Solid Edge part; units mm, degrees
sketch "Sketch1" plane through (0, 0, 0) normal (0, 0, 1) x (1, 0, 0)
  line L0 (-23.7579, 34.8421) -> (-23.7579, -27.1579)
  line L1 (-23.7579, -27.1579) -> (38.2421, -27.1579)
  line L2 (38.2421, -27.1579) -> (38.2421, 34.8421)
  line L3 (38.2421, 34.8421) -> (-23.7579, 34.8421)
  line L4 (-27.7579, 38.8421) -> (-27.7579, -31.1579)
  line L5 (-27.7579, -31.1579) -> (42.2421, -31.1579)
  line L6 (42.2421, -31.1579) -> (42.2421, 38.8421)
  line L7 (42.2421, 38.8421) -> (-27.7579, 38.8421)
  dimension "D1" = 42.2421
  dimension "D2" = 42.2421
  dimension "D3" = 38.2421
extrude "Protrusion1" add sketch "Sketch1" along normal blind 125
hole "Hole_1" at (-17.7579, 38.8421, 62.5) direction (0, -1, 0) diameter 7 end up to next
hole "Hole1" at (-17.7579, 38.8421, 25) direction (0, -1, 0) diameter 7 end up to next
hole "Hole2" at (-17.7579, 38.8421, 100) direction (0, -1, 0) diameter 7 end up to next
hole "Hole_4" at (-12.7579, -31.1579, 62.5) direction (0, 1, 0) diameter 7 end up to next
hole "Hole3" at (-12.7579, -31.1579, 100) direction (0, 1, 0) diameter 7 end up to next
hole "Hole4" at (27.2421, -31.1579, 100) direction (0, 1, 0) diameter 7 end up to next
hole "Hole5" at (27.2421, -31.1579, 62.5) direction (0, 1, 0) diameter 7 end up to next
hole "Hole6" at (27.2421, -31.1579, 25) direction (0, 1, 0) diameter 7 end up to next
hole "Hole7" at (-12.7579, -31.1579, 25) direction (0, 1, 0) diameter 7 end up to next
Geometry check sheet. Reference: the model listing, model coordinates, mm. A direction names the side the tool comes from. Coordinates: 2 decimals unless noted, no trailing zeros. Order: outer loops, then holes, each group sorted by start corner. A loop starts at its lowest first (then second) coordinate and runs counter-clockwise, first axis right, second up. Notation, with made-up numbers: M 74.25,28 L 109.25,28 A33 cw 109.25,63 Z; hole C 75,11 d5. An arc over 180 degrees is marked long. Answer as a JSON object with one key per item and string values.
Q1. Release check for a two-part mould opening along X. For faces 4 (the flat face through (-27.758, 4, 62)), 5 (the cylindrical face through (-11.71, -29.19, 96.66)), 6 (the flat face through (8, 38.842, 62)) record: released by +X, released by -X, zero draft, split by the parting line, or undercut.
Results are:
{"face 4": "released by -X", "face 5": "undercut", "face 6": "zero draft"}
Q2. Cross-section at A-A on z = 62.5. Record the cut outline in (x, y), and give its area (3 significant figures).
Results are:
{"outline": "M -27.76,-31.16 L -16.26,-31.16 L -16.26,-27.16 L -23.76,-27.16 L -23.76,34.84 L -21.26,34.84 L -21.26,38.84 L -27.76,38.84 Z; M -14.26,34.84 L 38.24,34.84 L 38.24,-27.16 L 30.74,-27.16 L 30.74,-31.16 L 42.24,-31.16 L 42.24,38.84 L -14.26,38.84 Z; M -9.26,-31.16 L 23.74,-31.16 L 23.74,-27.16 L -9.26,-27.16 Z", "area": "972 mm²"}
Q3. Cross-section at B-B on y = -11.5. Record the cut outline in (x, z), and give its area (4 significant figures).
Results are:
{"outline": "M -27.76,0 L -23.76,0 L -23.76,125 L -27.76,125 Z; M 38.24,0 L 42.24,0 L 42.24,125 L 38.24,125 Z", "area": "1,000 mm²"}
Q4. Cross-section at D-D on z = 75.5. Record the cut outline in (x, y), and give its area (3 significant figures).
Results are:
{"outline": "M -27.76,-31.16 L 42.24,-31.16 L 42.24,38.84 L -27.76,38.84 Z; hole M -23.76,-27.16 L 38.24,-27.16 L 38.24,34.84 L -23.76,34.84 Z", "area": "1,060 mm²"}
Q5. Depth check by flat-ended pin: pin 1 Ø6.5 at (x, z) = (27.24, 62.5) entering from -Y; pin 2 Ø4 at (x, z) = (-17.76, 25) entering from +Y. Enter the tip coordinate at first touch or a pass-through.
Results are:
{"pin 1": "stops at y = 34.84", "pin 2": "stops at y = -27.16"}
Q6. Tool access check on faces 1 (the flat face through (38.242, 3, 62)), 2 (the cylindrical face through (-17.604, 36.87, 59.003)), 3 (the cylindrical face through (-9.807, -29.186, 23.118)). Record the directions out of +Z, -Z, +X, -X, +Y, -Y that give a thin tool (end or side, any length) a straight path to the whole face; none if there is none.
Results are:
{"face 1": "+Z, -Z", "face 2": "+Y", "face 3": "-Y"}
Q7. Scan lines: line 1 (X direction, y = -29.6, z = 100); line 2 (X direction, y = -10.5, z = 63); line 3 (Y direction, x = -4.5, z = 18). Record each from-to range of solid material in increasing order.
Results are:
{"line 1": "x = -27.76 to -16.26, -9.26 to 23.74, 30.74 to 42.24", "line 2": "x = -27.76 to -23.76, 38.24 to 42.24", "line 3": "y = -31.16 to -27.16, 34.84 to 38.84"}
Q8. Cross-section at C-C on x = 7.5. Record the cut outline in (y, z), and give its area (3 significant figures).
Results are:
{"outline": "M -31.16,0 L -27.16,0 L -27.16,125 L -31.16,125 Z; M 34.84,0 L 38.84,0 L 38.84,125 L 34.84,125 Z", "area": "1,000 mm²"}
